from build123d import *

# Parameters (mm, degrees)
BOX_W           = 35
BOX_H           = 40
BOX_DEPTH       = 5
PAD_DEPTH       = 35
SKETCH001_R     = 6.05
POCKET_DEPTH    = 35.001
SKETCH002_R     = 1.65
POCKET001_DEPTH = 15.651
SKETCH003_R     = 2.9
POCKET002_DEPTH = 3
CHAMFER_SIZE    = 1
CHAMFER001_SIZE = 1


with BuildPart() as part:
    # Box → Box (new body)
    with BuildSketch(Plane.XY):
        with Locations((17.5, 20)):
            Rectangle(BOX_W, BOX_H)
    extrude(amount=BOX_DEPTH)

    # Sketch → Pad (new body)
    with BuildSketch(Plane.YZ.offset(35)):
        with BuildLine():
            ThreePointArc((14.906847, 11.265317), (24.712853, 4.206385), (15.722004, 12.277996))
            Line((15.722004, 12.277996), (14.590633, 13.409367))
            ThreePointArc((27.65, 7.999994), (22.927531, 15.067677), (14.590633, 13.409367))
            Line((27.65, 7.999994), (27.65, 0))
            Line((12.35, 0), (27.65, 0))
            Line((12.35, 0), (12.35, 7.999994))
            ThreePointArc((13.559898, 12.128872), (12.658702, 10.151243), (12.35, 7.999994))
            Line((13.559898, 12.128872), (14.906847, 11.265317))
        make_face()
    extrude(amount=-PAD_DEPTH)

    # Sketch001 → Pocket (cut, through all)
    with BuildSketch(Plane.YZ.offset(35)):
        with Locations((20, 8)):
            Circle(SKETCH001_R)
    extrude(amount=-POCKET_DEPTH, mode=Mode.SUBTRACT)

    # Sketch002 → Pocket001 (cut, through all)
    with BuildSketch(Plane(origin=(0, 0, 0), x_dir=(1, 0, 0), z_dir=(0, 0, -1))):
        with Locations((6.75, -6)):
            Circle(SKETCH002_R)
        with Locations((28.25, -6)):
            Circle(SKETCH002_R)
        with Locations((6.75, -34)):
            Circle(SKETCH002_R)
        with Locations((28.25, -34)):
            Circle(SKETCH002_R)
    extrude(amount=-POCKET001_DEPTH, mode=Mode.SUBTRACT)

    # Sketch003 → Pocket002 (cut)
    with BuildSketch(Plane.XY.offset(5)):
        with Locations((6.75, 34)):
            Circle(SKETCH003_R)
        with Locations((28.25, 34)):
            Circle(SKETCH003_R)
        with Locations((6.75, 6)):
            Circle(SKETCH003_R)
        with Locations((28.25, 6)):
            Circle(SKETCH003_R)
    extrude(amount=-POCKET002_DEPTH, mode=Mode.SUBTRACT)

    # Chamfer
    chamfer_edges = [part.edges().sort_by_distance(p)[0] for p in [
        (35, 20, 1.95),
    ]]
    chamfer(chamfer_edges, length=CHAMFER_SIZE)

    # Chamfer001
    chamfer001_edges = [part.edges().sort_by_distance(p)[0] for p in [
        (0, 20, 1.95),
    ]]
    chamfer(chamfer001_edges, length=CHAMFER001_SIZE)


solid = part.part
The model under review builds one solid part; all positions refer to its coordinate system, in mm. A direction names the side the tool comes from. Give positions to 0.01 mm unless a question says otherwise; leave off trailing zeros. Order: outer loops, then holes, each group sorted by start corner. A loop starts at its lowest first (then second) coordinate and runs counter-clockwise, first axis right, second up. Notation, with made-up numbers: (37.25, -24.75) -> (86.25, -24.75) arc R29 cw to (86.25, -1.75) -> close; hole circle Ø3 at (73.25, 42). An arc over 180 degrees is marked (long way). Write item = value, one per line. Start each with the question number.
(1) Take a section at A-A (y = 6). Write out the cut boundary in (x, z), plus the area to 3 significant figures.
(2) Take a section at B-B (x = 6.75). State how many separate pieces and enclosed holes the cut face has, plus the area to 3 significant figures.
(3) Take a section at C-C (y = 20). Write out the cut boundary in (x, z), plus the area to 3 significant figures.
(4) Draft analysis for pull direction X (two halves, no side actions). For faces 5 (the flat face through (17, 40, 2)), 6 (the cylindrical face through (26.94, 7, 0.99)), 7 (the flat face through (0, 20.1, 0.3)), 8 (the cylindrical face through (30.93, 32.89, 3.52)), state which applies: +X half, -X half, draft (parallel to the pull), parting line (faces both ways), or undercut.
(5) Tool access review of faces 1 (the cylindrical face through (4.449, 32.235, 3.521)), 2 (the flat face through (17, 6, 5)), 3 (the flat face through (18, 27.65, 7)), 4 (the cylindrical face through (17.731, 13.953, 8.201)): name each direction out of +Z, -Z, +X, -X, +Y, -Y from which nothing blocks a thin tool from reaching the whole face with its end or side.
(6) For pin 1 Ø6.5 at (x, y) = (27.5, 33.5) entering from +Z; pin 2 Ø0.9 at (x, z) = (11, 6) entering from +Y; pin 3 Ø3 at (x, y) = (22.5, 12.5) entering from +Z, all flat-tipped, find the tip position at first contact; note any pin that passes through.
(7) For L1, parallel to Y at x = 6.75, z = 0.8; L2, parallel to X at y = 6, z = 1.45; L3, parallel to Z at x = 18, y = 20, list the stretches that pass through material, from the lowest coordinate up. Write a range as from..to.
Returned:
q1.outline = (0, 0) -> (5.1, 0) -> (5.1, 2) -> (3.85, 2) -> (3.85, 5) -> (0, 5) -> close; (8.4, 0) -> (26.6, 0) -> (26.6, 2) -> (25.35, 2) -> (25.35, 5) -> (9.65, 5) -> (9.65, 2) -> (8.4, 2) -> close; (29.9, 0) -> (35, 0) -> (35, 5) -> (31.15, 5) -> (31.15, 2) -> (29.9, 2) -> close
q1.area = 127 mm²
q2.separate_pieces = 3
q2.enclosed_holes = 0
q2.area = 172 mm²
q3.outline = (0, 0) -> (35, 0) -> (35, 0.95) -> (34, 1.95) -> (1, 1.95) -> (0, 0.95) -> close; (0, 15.05) -> (1, 14.05) -> (34, 14.05) -> (35, 15.05) -> (35, 15.65) -> (0, 15.65) -> close
q3.area = 122 mm²
q4.face_5 = draft
q4.face_6 = undercut
q4.face_7 = -X half
q4.face_8 = undercut
q5.face_1 = +Z
q5.face_2 = +Z, +X, -X, -Y
q5.face_3 = +Z, +X, -X, +Y
q5.face_4 = +X, -X
q6.pin_1 = 5
q6.pin_2 = 27.65
q6.pin_3 = 12.13
q7.L1 = 0..4.35, 7.65..32.35, 35.65..40
q7.L2 = 0..5.1, 8.4..26.6, 29.9..35
q7.L3 = 0..1.95, 14.05..15.65
